Geometry check sheet. Reference: the model listing, model coordinates, mm. A direction names the side the tool comes from. Give positions to 0.01 mm unless a question says otherwise; leave off trailing zeros. Write each loop counter-clockwise with the first axis right and the second up, starting at its lowest first coordinate (ties: lowest second). Pieces come first, ordered by that corner, then holes.
(1) Cross-section at C-C (y = -0.7). Count the separate pieces of the cut face and the enclosed holes in it, and give its area (3 significant figures).
(2) Cross-section at B-B (x = 18.5). Record the boundary of the cut face in (y, z), and give its area (3 significant figures).
(3) Cross-section at A-A (z = 6). Record the boundary of the cut face in (x, y).
(4) Depth check by flat-ended pin: P1, Ø3, axis at x = 14, z = 1.5, coming from the +Y side; P2, Ø0.6, axis at x = 2, z = 5.5, coming from the -Y side; P3, Ø6, axis at x = 9, z = 6, coming from the +Y side. Enter the tip coordinate at first touch or a pass-through.
(5) Thickness scan on line 1 along X through (y, z) = (0.3, 1.5); line 2 along X through (y, z) = (1.4, 1.75); line 3 along Z through (x, y) = (9, 1.85). Record the ranges inside material, lowest first.
(6) Mould release check, pull along X, two halves, no side actions. Record for faces 4 (the flat face through (9.9, 3, 0.6)), 5 (the flat face through (20, 1, 6)), 6 (the cylindrical face through (13.024, 0.378, 1.283)): +X half, -X half, draft (parallel to the pull), parting line (faces both ways), or undercut.
(7) Tool access check on faces 1 (the flat face through (10, 1, 12)), 2 (the cylindrical face through (4, 2, 6)), 3 (the cylindrical face through (1.4, 0.4, 5.2)). Record the directions out of +Z, -Z, +X, -X, +Y, -Y that give a thin tool (end or side, any length) a straight path to the whole face; none if there is none.
```python
from build123d import *

# Parameters (mm, degrees)
SKETCH_1_W               = 20
SKETCH_1_H               = 12
EXTRUDE_1_DEPTH          = 3
EXTRUDE_3_DEPTH          = 1.3
EXTRUDE_3_DEPTH_BACK     = 1.2
SKETCH_1_13_W            = 20
SKETCH_1_13_H            = 12
SKETCH_1_13_R            = 2.6
SKETCH_1_13_R_2          = 3
EXTRUDE_START            = -1.2
SKETCH_1_14_W            = 20
SKETCH_1_14_H            = 12
SKETCH_1_14_R            = 2.6
EXTRUDE_4_DEPTH          = 1.2
CUT_EXTRUDE_3_DEPTH      = 24.515952033
CUT_EXTRUDE_3_DEPTH_BACK = 24.515952033
SKETCH_3_R               = 0.75
SKETCH_3_R_2             = 0.35
CUT_EXTRUDE_START        = -1.2
SKETCH_3_4_R             = 1
CUT_EXTRUDE_4_DEPTH      = 3.2


with BuildPart() as part:
    # 草图1 → 凸台-拉伸1 (new body)
    with BuildSketch(Plane(origin=(0, 0, 0), x_dir=(1, 0, 0), z_dir=(0, 1, 0))):
        with Locations((10, -6)):
            Rectangle(SKETCH_1_W, SKETCH_1_H)
        with BuildLine():
            ThreePointArc((13.333333333, -3.505561742), (18, -6), (13.333333333, -8.494438258))
            ThreePointArc((13.333333333, -8.494438258), (4, -6), (13.333333333, -3.505561742))
        make_face(mode=Mode.SUBTRACT)
    extrude(amount=EXTRUDE_1_DEPTH)

    # 草图1<13> → 凸台-拉伸3 (add, two sides: drawn at the far end of the back side and taken through both)
    with BuildSketch(Plane(origin=(0, 0, 0), x_dir=(1, 0, 0), z_dir=(0, 1, 0)).offset(-EXTRUDE_3_DEPTH_BACK)):
        with Locations((10, -6)):
            Rectangle(SKETCH_1_13_W, SKETCH_1_13_H)
        with Locations(Location((9, -6, 0), (0, 0, 270))):
            Circle(SKETCH_1_13_R, mode=Mode.SUBTRACT)
        with Locations(Location((15, -6, 0), (0, 0, 123.748988596))):
            Circle(SKETCH_1_13_R_2, mode=Mode.SUBTRACT)
    extrude(amount=EXTRUDE_3_DEPTH + EXTRUDE_3_DEPTH_BACK)

    # 草图1<14> → 凸台-拉伸4 (add)
    with BuildSketch(Plane(origin=(0, 0, 0), x_dir=(1, 0, 0), z_dir=(0, 1, 0)).offset(EXTRUDE_START)):
        with Locations((10, -6)):
            Rectangle(SKETCH_1_14_W, SKETCH_1_14_H)
        with Locations(Location((15, -6, 0), (0, 0, 270))):
            Circle(SKETCH_1_14_R, mode=Mode.SUBTRACT)
        with Locations(Location((9, -6, 0), (0, 0, 270))):
            Circle(SKETCH_1_14_R, mode=Mode.SUBTRACT)
    extrude(amount=EXTRUDE_4_DEPTH)

    # 草图3 → 切除-拉伸3 (cut, two sides: drawn at the far end of the back side and taken through both)
    with BuildSketch(Plane(origin=(0, 0, 0), x_dir=(1, 0, 0), z_dir=(0, 1, 0)).offset(-CUT_EXTRUDE_3_DEPTH_BACK)):
        with Locations(Location((2, -6, 0), (0, 0, 270))):
            Circle(SKETCH_3_R)
        with Locations(Location((14, -1.5, 0), (0, 0, 270))):
            Circle(SKETCH_3_R)
        with Locations(Location((14, -10.5, 0), (0, 0, 270))):
            Circle(SKETCH_3_R)
        with Locations(Location((1.5, -1.5, 0), (0, 0, 270))):
            Circle(SKETCH_3_R_2)
        with Locations(Location((18.5, -1.5, 0), (0, 0, 270))):
            Circle(SKETCH_3_R_2)
        with Locations(Location((1.5, -10.5, 0), (0, 0, 270))):
            Circle(SKETCH_3_R_2)
        with Locations(Location((18.5, -10.5, 0), (0, 0, 270))):
            Circle(SKETCH_3_R_2)
    extrude(amount=CUT_EXTRUDE_3_DEPTH + CUT_EXTRUDE_3_DEPTH_BACK, mode=Mode.SUBTRACT)

    # 草图3<4> → 切除-拉伸4 (cut)
    with BuildSketch(Plane(origin=(0, 0, 0), x_dir=(1, 0, 0), z_dir=(0, 1, 0)).offset(CUT_EXTRUDE_START)):
        with Locations(Location((2, -6, 0), (0, 0, 270))):
            Circle(SKETCH_3_4_R)
        with Locations(Location((14, -1.5, 0), (0, 0, 270))):
            Circle(SKETCH_3_4_R)
        with Locations(Location((14, -10.5, 0), (0, 0, 270))):
            Circle(SKETCH_3_4_R)
    extrude(amount=CUT_EXTRUDE_4_DEPTH, mode=Mode.SUBTRACT)


solid = part.part
```
Reply:
1. separate pieces: 1
1. enclosed holes: 9
1. area: 187 mm2
2. outline: (-1.2, 0) - (3, 0) - (3, 1.15) - (-1.2, 1.15) - close; (-1.2, 1.85) - (3, 1.85) - (3, 10.15) - (-1.2, 10.15) - close; (-1.2, 10.85) - (3, 10.85) - (3, 12) - (-1.2, 12) - close
2. area: 44.5 mm2
3. outline: (0, -1.2) - (1, -1.2) - (1, 2) - (1.25, 2) - (1.25, 3) - (0, 3) - close; (2.75, 2) - (3, 2) - (3, -1.2) - (6.4, -1.2) - (6.4, 1.3) - (4, 1.3) - (4, 3) - (2.75, 3) - close; (11.6, -1.2) - (12.4, -1.2) - (12.4, 0) - (12, 0) - (12, 1.3) - (11.6, 1.3) - close; (17.6, -1.2) - (20, -1.2) - (20, 3) - (18, 3) - (18, 0) - (17.6, 0) - close
4. P1: stops at y = 3
4. P2: stops at y = 2
4. P3: stops at y = 1.3
5. line 1: x = 0 to 1.15, 1.85 to 13, 15 to 18.15, 18.85 to 20
5. line 2: x = 0 to 1.26, 1.74 to 6.37, 11.63 to 13.03, 14.97 to 18.26, 18.74 to 20
5. line 3: z = 0 to 1, 11 to 12
6. face 4: draft
6. face 5: +X half
6. face 6: undercut
7. face 1: +Z, +X, -X, +Y, -Y
7. face 2: +Y
7. face 3: -Y
